```python
from build123d import *

# Parameters (mm, degrees)
F1_DEPTH = 0.635


with BuildPart() as f1:
    # F0 (on Front) → F1 (new body, symmetric)
    with BuildSketch(Plane.XZ):
        with BuildLine():
            Line((-0.635, 7.47181), (-0.635, 9.50381))
            ThreePointArc((-0.635, 9.50381), (-6.735192, 6.735192), (-9.50381, 0.635))
            Line((-9.50381, 0.635), (-7.47181, 0.635))
            Line((-7.47181, 0.635), (-7.47181, -0.635))
            Line((-7.47181, -0.635), (-9.50381, -0.635))
            ThreePointArc((-9.50381, -0.635), (-6.735192, -6.735192), (-0.635, -9.50381))
            Line((-0.635, -9.50381), (-0.635, -7.47181))
            Line((-0.635, -7.47181), (0.635, -7.47181))
            Line((0.635, -7.47181), (0.635, -9.50381))
            ThreePointArc((0.635, -9.50381), (6.735192, -6.735192), (9.50381, -0.635))
            Line((9.50381, -0.635), (7.47181, -0.635))
            Line((7.47181, -0.635), (7.47181, 0.635))
            Line((7.47181, 0.635), (9.50381, 0.635))
            ThreePointArc((9.50381, 0.635), (6.735192, 6.735192), (0.635, 9.50381))
            Line((0.635, 9.50381), (0.635, 7.47181))
            Line((0.635, 7.47181), (-0.635, 7.47181))
        make_face()
    extrude(amount=F1_DEPTH, both=True)


solid = f1.part
```
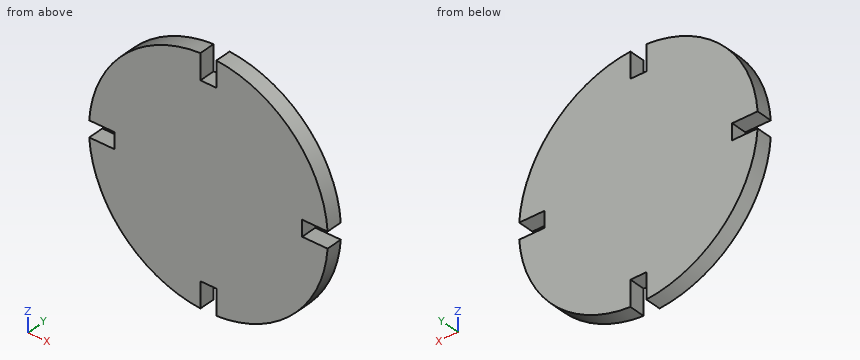
CAD build for the part. Positions are in the model's coordinates, mm. Give positions to 0.01 mm unless a question says otherwise; leave off trailing zeros. Loops run counter-clockwise (first coordinate to the right, second up) from the corner with the lowest first, then second, coordinate; pieces in that order, holes last. Notation, with made-up numbers: (44, 2) - (83, 2) arc R29 ccw to (83, 26) - close; hole circle Ø4 at (86, -18.5). An arc over 180 degrees is marked (long way). Put each result on its own line as item: value.
Q1. Slice it at B-B (y = 0). Give the cut face in (x, z) (3 decimals), plus the area to 3 significant figures.
Filled in:
outline: (-9.504, -0.635) arc R9.525 ccw to (-0.635, -9.504) - (-0.635, -7.472) - (0.635, -7.472) - (0.635, -9.504) arc R9.525 ccw to (9.504, -0.635) - (7.472, -0.635) - (7.472, 0.635) - (9.504, 0.635) arc R9.525 ccw to (0.635, 9.504) - (0.635, 7.472) - (-0.635, 7.472) - (-0.635, 9.504) arc R9.525 ccw to (-9.504, 0.635) - (-7.472, 0.635) - (-7.472, -0.635) - close
area: 275 mm²
Q2. Slice it at A-A (x = -7.75). Give the cut face in (y, z) (3 decimals).
Filled in:
outline: (-0.635, -5.537) - (0.635, -5.537) - (0.635, -0.635) - (-0.635, -0.635) - close; (-0.635, 0.635) - (0.635, 0.635) - (0.635, 5.537) - (-0.635, 5.537) - close
Q3. Probe line 1 along X through (y, z) = (0.6, -0.5); line 2 along X through (y, z) = (0.5, -8) (3 decimals); line 3 along X through (y, z) = (0.35, -8.25) (3 decimals). List the from-to ranges inside material, lowest first.
Filled in:
line 1: x = -7.47 to 7.47
line 2: x = -5.17 to -0.635, 0.635 to 5.17
line 3: x = -4.761 to -0.635, 0.635 to 4.761
Q4. Flat gauge pins, fed straight in: pin 1 (0.6 mm diameter, centred on x = 0, y = 0.5, fed in from -Z); pin 2 (0.6 mm diameter, centred on y = 0, z = 0, fed in from -X); pin 3 (0.6 mm diameter, centred on x = 9, y = 0, fed in from +Z). Where does each tip first touch, or does it go through?
Filled in:
pin 1: stops at z = -7.47
pin 2: stops at x = -7.47
pin 3: stops at z = 3.88
Q5. Slice it at C-C (x = 6.5). Give the cut face in (y, z) (3 decimals).
Filled in:
outline: (-0.635, -6.962) - (0.635, -6.962) - (0.635, 6.962) - (-0.635, 6.962) - close
Q6. Slice it at D-D (z = 7). Give the cut face in (x, y) (3 decimals), plus the area to 3 significant figures.
Filled in:
outline: (-6.46, -0.635) - (6.46, -0.635) - (6.46, 0.635) - (-6.46, 0.635) - close
area: 16.4 mm²
